Source: CAD feature listing. Evaluate the final solid. Frame: model axes, mm. A direction names the side the tool comes from. Coordinates: 2 decimals unless noted, no trailing zeros. Write each loop counter-clockwise with the first axis right and the second up, starting at its lowest first coordinate (ties: lowest second). Pieces come first, ordered by that corner, then holes. Notation, with made-up numbers: M 75,28.5 L 115,28.5 A23 cw 115,45.5 Z; hole C 86,11 d9. An arc over 180 degrees is marked long. One line per item, written item: value. Start each with the question number.
Item 1: Pin query (flat end, axial travel): P1, Ø4, axis at y = -8, z = 3, coming from the +X side; P2, Ø1.5, axis at x = -2.5, y = 2, coming from the +Z side. Return the tip coordinate at first contact, or that it passes through.
Item 2: Ray query, L1, parallel to Z at x = 5, y = 3.5; L2, parallel to X at y = -7.25, z = 4.75; L3, parallel to Y at x = 5.2, z = 3. Return the intervals inside material, ascending. Write a range as from..to.
Item 3: Cut plane B-B, the plane x = 9.75. Output: boundary loops of the cut face in (y, z), then the cut area to 3 significant figures.
Item 4: Cut plane D-D, the plane x = 0. Output: boundary loops of the cut face in (y, z), then the cut area to 3 significant figures.
Item 5: Mould query, pull axis Z, two halves, no side actions, for faces 5 (the cylindrical face through (5.014, -9.582, 0.937)), 6 (the flat face through (4, -8, 3)), 7 (the flat face through (0, 0, 0)), 8 (the flat face through (-11, 0, 3)). Classes: released by +Z, released by -Z, zero draft, split by the parting line, or undercut.
Item 6: Cut plane A-A, the plane z = 3. Output: boundary loops of the cut face in (x, y).
Item 7: Set-up query: faces 1 (the cylindrical face through (5.01, 5.46, 2.44)), 2 (the cylindrical face through (-5.158, -3.955, 3.944)), 3 (the flat face through (0, 0, -2)), 4 (the cylindrical face through (8.54, 5.56, 2.46)). Return all of +Z, -Z, +X, -X, +Y, -Y with unobstructed straight access to the full face (end or side cutting, diameter ignored); none if empty.
Item 8: Cut plane C-C, the plane y = -8. Output: boundary loops of the cut face in (x, z), then the cut area to 3 significant figures.
```python
from build123d import *

# Parameters (mm, degrees)
CYLINDER095_R          = 2.6
CYLINDER095_DEPTH      = 2
CYLINDER096_R          = 2.5
CYLINDER096_DEPTH      = 5
CYLINDER094_R          = 6.5
CYLINDER094_DEPTH      = 130
CYLINDER098_R          = 2.6
CYLINDER098_DEPTH      = 2
CYLINDER097_R          = 2.5
CYLINDER097_DEPTH      = 5
BOX026_W               = 10
BOX026_H               = 22
BOX026_DEPTH           = 22
CUT053_PLACEMENT_ANGLE = 90


with BuildPart() as cilindro095:
    # Cylinder095 → Cylinder095 (new body)
    with BuildSketch(Plane.XY.offset(5)):
        Circle(CYLINDER095_R)
    extrude(amount=CYLINDER095_DEPTH)


with BuildPart() as obj1:
    # Cylinder096 → Cylinder096 (new body)
    with BuildSketch(Plane.XY):
        Circle(CYLINDER096_R)
    extrude(amount=CYLINDER096_DEPTH)

    # Fusion036: union Cilindro095
    add(cilindro095.part)


with BuildPart() as obj1_1:
    # Fusion036 placement: moved
    add(obj1.part.moved(Location((3, 8, -11))))


with BuildPart() as cilindro094:
    # Cylinder094 → Cylinder094 (new body)
    with BuildSketch(Plane(origin=(0, 0, 0), x_dir=(0, 0, -1), z_dir=(1, 0, 0))):
        Circle(CYLINDER094_R)
    extrude(amount=CYLINDER094_DEPTH)


with BuildPart() as cilindro098:
    # Cylinder098 → Cylinder098 (new body)
    with BuildSketch(Plane.XY.offset(5)):
        Circle(CYLINDER098_R)
    extrude(amount=CYLINDER098_DEPTH)


with BuildPart() as fusion038:
    # Cylinder097 → Cylinder097 (new body)
    with BuildSketch(Plane.XY):
        Circle(CYLINDER097_R)
    extrude(amount=CYLINDER097_DEPTH)

    # Fusion037: union Cilindro098
    add(cilindro098.part)


with BuildPart() as fusion038_1:
    # Fusion037 placement: moved
    add(fusion038.part.moved(Location((3, -8, -11))))

    # Fusion038: union obj1, Cilindro094
    add(obj1_1.part)
    add(cilindro094.part)


with BuildPart() as obj2:
    # Box026 → Box026 (new body)
    with BuildSketch(Plane(origin=(-2, -11, -11), x_dir=(1, 0, 0), z_dir=(0, 0, 1))):
        with Locations((5, 11)):
            Rectangle(BOX026_W, BOX026_H)
    extrude(amount=BOX026_DEPTH)

    # Cut053: cut Fusion038
    add(fusion038_1.part, mode=Mode.SUBTRACT)


with BuildPart() as obj2_1:
    # Cut053 placement: moved
    add(obj2.part.rotate(Axis((0, 0, 0), (0, -1, 0)), CUT053_PLACEMENT_ANGLE))


solid = obj2_1.part
```
From the geometry:
1. P1: stops at x = 4
1. P2: stops at z = 0
2. L1: z = -2..0
2. L2: x = -11..4
2. L3: y = -11..-10.6, -5.4..-3.9, 3.9..5.4, 10.6..11
3. outline: M -11,-2 L 11,-2 L 11,8 L -11,8 Z; hole C -8,3 d5; hole C 8,3 d5
3. area: 181 mm²
4. outline: M -11,-2 L 11,-2 L 11,8 L 6.5,8 L 6.5,0 L -6.5,0 L -6.5,8 L -11,8 Z
4. area: 116 mm²
5. face 5: undercut
5. face 6: undercut
5. face 7: released by +Z
5. face 8: zero draft
6. outline: M -11,-11 L 11,-11 L 11,-10.5 L 6,-10.5 L 6,-10.6 L 4,-10.6 L 4,-5.4 L 6,-5.4 L 6,-5.5 L 11,-5.5 L 11,5.5 L 6,5.5 L 6,5.4 L 4,5.4 L 4,10.6 L 6,10.6 L 6,10.5 L 11,10.5 L 11,11 L -11,11 Z; hole C 0,0 d13
7. face 1: none
7. face 2: +Z
7. face 3: -Z, +X, -X, +Y, -Y
7. face 4: +X
8. outline: M -11,-2 L 11,-2 L 11,0.5 L 6,0.5 L 6,0.4 L 4,0.4 L 4,5.6 L 6,5.6 L 6,5.5 L 11,5.5 L 11,8 L -11,8 Z
8. area: 185 mm²
